Could you check a few things on this model? Use its own coordinates, in mm. Face numbers are marked on the shaded views. A direction names the side the tool comes from. Give positions to 0.01 mm unless a question says otherwise; leave off trailing zeros. Order: outer loops, then holes, each group sorted by start corner. A loop starts at its lowest first (then second) coordinate and runs counter-clockwise, first axis right, second up. Notation, with made-up numbers: (5.5, 58.25) -> (29.5, 58.25) arc R17 ccw to (29.5, 78.25) -> close; hole circle Ø4 at (34.5, 85.25). An arc over 180 degrees is marked (long way). Write each question's results on one line, items separated by ' | '.
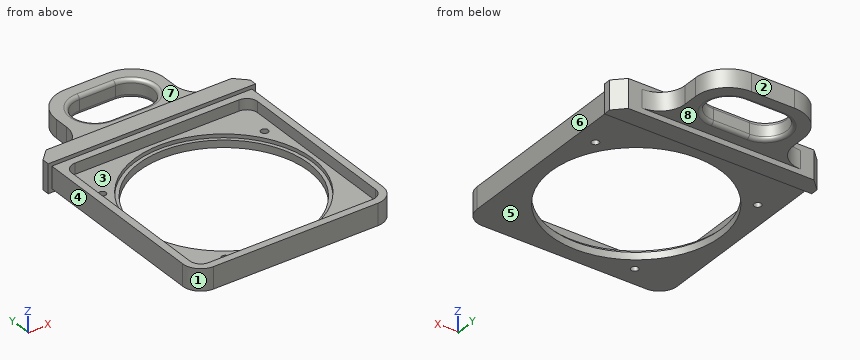
```python
from build123d import *

# Parameters (mm, degrees)
SKETCH_W        = 55.5
SKETCH_H        = 55.5
SKETCH_R        = 24.6
PAD_DEPTH       = 6
SKETCH001_W     = 57.5
SKETCH001_H     = 8
PAD001_DEPTH    = 5
SKETCH002_W     = 30
SKETCH002_H     = 5
PAD002_DEPTH    = 20
FILLET_R        = 5
POCKET_DEPTH    = 6
FILLET001_R     = 9
FILLET002_R     = 7
CHAMFER_SIZE    = 3
SKETCH004_R     = 24.6
SKETCH004_R_2   = 23.6
PAD003_DEPTH    = 2
SKETCH005_W     = 51.5
SKETCH005_H     = 51.5
POCKET001_DEPTH = 3
SKETCH006_R     = 1
POCKET002_DEPTH = 6
FILLET003_R     = 1
FILLET004_R     = 1
FILLET005_R     = 3


with BuildPart() as part:
    # Sketch → Pad (new body)
    with BuildSketch(Plane.XY):
        Rectangle(SKETCH_W, SKETCH_H)
        Circle(SKETCH_R, mode=Mode.SUBTRACT)
    extrude(amount=PAD_DEPTH)

    # Sketch001 → Pad001 (new body)
    with BuildSketch(Plane(origin=(0, 27.75, 0), x_dir=(-1, 0, 0), z_dir=(0, 1, 0))):
        with Locations((0, 3)):
            Rectangle(SKETCH001_W, SKETCH001_H)
    extrude(amount=PAD001_DEPTH)

    # Sketch002 → Pad002 (new body)
    with BuildSketch(Plane(origin=(0, 32.75, 0), x_dir=(-1, 0, 0), z_dir=(0, 1, 0))):
        with Locations((0, 3)):
            Rectangle(SKETCH002_W, SKETCH002_H)
    extrude(amount=PAD002_DEPTH)

    # Fillet
    fillet_edges = [part.edges().sort_by_distance(p)[0] for p in [
        (-27.75, -27.75, 3),
        (27.75, -27.75, 3),
    ]]
    fillet(fillet_edges, radius=FILLET_R)

    # Sketch003 → Pocket (cut)
    with BuildSketch(Plane(origin=(0, 0, 0.5), x_dir=(1, 0, 0), z_dir=(0, 0, -1))):
        with BuildLine():
            ThreePointArc((-5, -36.75), (-11, -42.75), (-5, -48.75))
            Line((-5, -48.75), (5, -48.75))
            ThreePointArc((5, -48.75), (11, -42.75), (5, -36.75))
            Line((-5, -36.75), (5, -36.75))
        make_face()
    extrude(amount=-POCKET_DEPTH, mode=Mode.SUBTRACT)

    # Fillet001
    fillet001_edges = [part.edges().sort_by_distance(p)[0] for p in [
        (15, 52.75, 3),
        (-15, 52.75, 3),
    ]]
    fillet(fillet001_edges, radius=FILLET001_R)

    # Fillet002
    fillet002_edges = [part.edges().sort_by_distance(p)[0] for p in [
        (15, 32.75, 3),
        (-15, 32.75, 3),
    ]]
    fillet(fillet002_edges, radius=FILLET002_R)

    # Chamfer
    chamfer_edges = [part.edges().sort_by_distance(p)[0] for p in [
        (-28.75, 32.75, 3),
        (28.75, 32.75, 3),
    ]]
    chamfer(chamfer_edges, length=CHAMFER_SIZE)

    # Sketch004 → Pad003 (new body)
    with BuildSketch(Plane(origin=(0, 0, 0), x_dir=(1, 0, 0), z_dir=(0, 0, -1))):
        Circle(SKETCH004_R)
        Circle(SKETCH004_R_2, mode=Mode.SUBTRACT)
    extrude(amount=-PAD003_DEPTH)

    # Sketch005 → Pocket001 (cut)
    with BuildSketch(Plane.XY.offset(6)):
        Rectangle(SKETCH005_W, SKETCH005_H)
    extrude(amount=-POCKET001_DEPTH, mode=Mode.SUBTRACT)

    # Sketch006 → Pocket002 (cut)
    with BuildSketch(Plane.XY.offset(3)):
        with Locations((-22.5, 15.549035)):
            Circle(SKETCH006_R)
        with Locations((22.5, 15.549035)):
            Circle(SKETCH006_R)
        with Locations((-15.687316, -22.403808)):
            Circle(SKETCH006_R)
    extrude(amount=-POCKET002_DEPTH, mode=Mode.SUBTRACT)

    # Fillet003
    fillet003_edges = [part.edges().sort_by_distance(p)[0] for p in [
        (0, 48.75, 5.5),
    ]]
    fillet(fillet003_edges, radius=FILLET003_R)

    # Fillet004
    fillet004_edges = [part.edges().sort_by_distance(p)[0] for p in [
        (0, 36.75, 0.5),
    ]]
    fillet(fillet004_edges, radius=FILLET004_R)

    # Fillet005
    fillet005_edges = [part.edges().sort_by_distance(p)[0] for p in [
        (-25.75, -25.75, 4.5),
        (25.75, -25.75, 4.5),
        (25.75, 25.75, 4.5),
        (-25.75, 25.75, 4.5),
    ]]
    fillet(fillet005_edges, radius=FILLET005_R)


solid = part.part
```
Q1. Suppose I cut it at B-B on x = 3. State how many separate pieces and enclosed holes the cut face has, and give its area (3 significant figures).
Here are the results:
separate pieces: 3 | enclosed holes: 0 | area: 115 mm²
Q2. Suppose I cut it at A-A on y = 42.75. Please give me the cut outline in (x, z), and give its area (3 significant figures).
Here are the results:
outline: (-15, 0.5) -> (-12, 0.5) arc R1 ccw to (-11, 1.5) -> (-11, 4.5) arc R1 ccw to (-12, 5.5) -> (-15, 5.5) -> close; (11, 1.5) arc R1 ccw to (12, 0.5) -> (15, 0.5) -> (15, 5.5) -> (12, 5.5) arc R1 ccw to (11, 4.5) -> close | area: 39.1 mm²
Q3. Suppose I cut it at D-D on y = 0. Please give me the cut outline in (x, z).
Here are the results:
outline: (-27.75, 0) -> (-23.6, 0) -> (-23.6, 2) -> (-24.6, 2) -> (-24.6, 3) -> (-25.75, 3) -> (-25.75, 6) -> (-27.75, 6) -> close; (23.6, 0) -> (27.75, 0) -> (27.75, 6) -> (25.75, 6) -> (25.75, 3) -> (24.6, 3) -> (24.6, 2) -> (23.6, 2) -> close
Q4. Suppose I cut it at C-C on x = -18. Please give me the cut outline in (y, z).
Here are the results:
outline: (-27.75, 0) -> (-15.26, 0) -> (-15.26, 2) -> (-16.77, 2) -> (-16.77, 3) -> (-25.75, 3) -> (-25.75, 6) -> (-27.75, 6) -> close; (15.26, 0) -> (27.75, 0) -> (27.75, -1) -> (32.75, -1) -> (32.75, 0.5) -> (34.01, 0.5) -> (34.01, 5.5) -> (32.75, 5.5) -> (32.75, 7) -> (27.75, 7) -> (27.75, 6) -> (25.75, 6) -> (25.75, 3) -> (16.77, 3) -> (16.77, 2) -> (15.26, 2) -> close
Q5. I need wall thicknesses on line 1 along Y through (x, z) = (-3, 4); line 2 along Y through (x, z) = (0, 0.6); line 3 along X through (y, z) = (-22, 5). Which ranges of each line are inside material? Lowest first, please.
Here are the results:
line 1: y = -27.75 to -25.75, 25.75 to 36.75, 48.75 to 52.75 | line 2: y = -27.75 to -23.6, 23.6 to 36.19, 49.31 to 52.75 | line 3: x = -27.75 to -25.75, 25.75 to 27.75
Q6. For the marked faces 4, 5, 6, 7 and 8, which set-ups out of +Z, -Z, +X, -X, +Y, -Y let a thin tool reach every point of the face, with its end or its side?
Here are the results:
face 4: +Z, -Z, -X, -Y | face 5: -Z, +X, -X, -Y | face 6: +Z, -Z, +X, -Y | face 7: +Z, +X, -X, +Y | face 8: -Z, +X, -X, +Y
Q7. I'm going to push flat-ended pins straight in: pin 1 Ø2 at (x, z) = (13.5, 4.5) entering from +Y; pin 2 Ø16 at (x, y) = (4.5, 44.5) entering from +Z; pin 3 Ø3 at (y, z) = (25.5, 2) entering from +X; pin 4 Ø1.2 at (x, y) = (22.5, 15.55) entering from -Z. Where does each tip first touch, or does it pass through?
Here are the results:
pin 1: stops at y = 49.97 | pin 2: stops at z = 5.5 | pin 3: stops at x = 27.75 | pin 4: passes through
Q8. Thinking about a two-plate mould opening in X: for the marked faces 1, 2 and 3, which applies, +X half, -X half, draft (parallel to the pull), parting line (faces both ways), or undercut?
Here are the results:
face 1: -X half | face 2: draft | face 3: undercut
